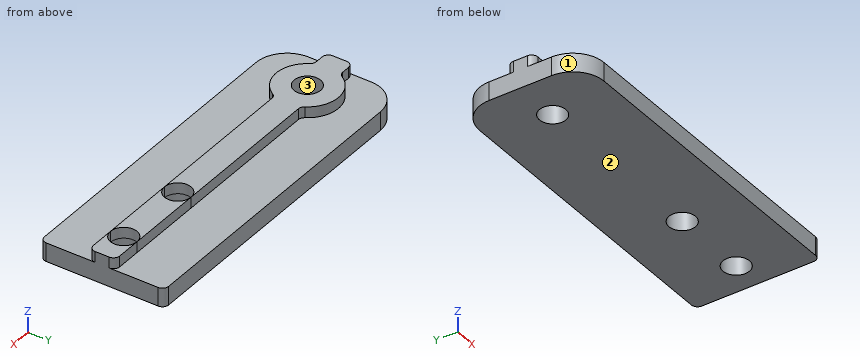
Autodesk Inventor part; units mm, degrees
ref_plane "YZ Plane" through (0, 0, 0) normal (1, 0, 0) x (0, 1, 0)
ref_plane "XZ Plane" through (0, 0, 0) normal (0, 1, 0) x (-1, 0, 0)
ref_plane "XY Plane" through (0, 0, 0) normal (0, 0, 1) x (1, 0, 0)
sketch "Szkic1" plane through (0, 0, 0) normal (0, 0, 1) x (1, 0, 0)
  line L0 (55, -20) -> (-55, -20)
  line L1 (-55, -20) -> (-55, 20)
  line L2 (-55, 20) -> (55, 20)
  line L3 (55, 20) -> (55, -20)
  line L4 (55, -20) -> (-55, 20) construction
  line L5 (-55, -20) -> (55, 20) construction
  line L6 (-55, 0) -> (55, 0) construction
  line L7 (-55, -4.25) -> (55, -4.25)
  line L8 (55, -4.25) -> (55, 4.25)
  line L9 (55, 4.25) -> (-55, 4.25)
  line L10 (-55, 4.25) -> (-55, -4.25)
  line L11 (-55, -4.25) -> (55, 4.25) construction
  line L12 (55, -4.25) -> (-55, 4.25) construction
  circle A0 centre (-40, 0) radius 10
  point P0 (0, 0)
  point P1 (0, 0)
  point P2 (-40, 0)
  point P3 (20, 0)
  point P4 (45, 0)
  dimension "d1" = 40
  dimension "d4" = 8.5
  dimension "d9" = 15
  dimension "d12" = 10
  dimension "d31" = 95
  dimension "d32" = 25
  dimension "d33" = 20
extrude "Wyciągnięcie proste1" add sketch "Szkic1" against normal blind 6
extrude "Wyciągnięcie proste2" add sketch "Szkic1" along normal blind 3.5 contours L7 A0 L9 L3 | L1 L9 A0 L7 | A0 L7 | L7 A0 L9 | L9 A0
fillet "Zaokrąglenie1" radius 2 10 edges at (55, 4.25, 1.75) (55, -4.25, 1.75) (55, 20, -3) (55, -20, -3) (-55, -4.25, 1.75) (-55, 4.25, 1.75) (-49.0519, -4.25, 1.75) (-30.9481, -4.25, 1.75) (-30.9481, 4.25, 1.75) (-49.0519, 4.25, 1.75)
fillet "Zaokrąglenie2" radius 10 2 edges at (-55, -20, -3) (-55, 20, -3)
hole "Otwór1" at (-40, 0, 0) at (20, 0, 0) at (45, 0, 0) direction (0, 0, -1) diameter 8.5 end through all
hole "Otwór2" at (45, 0, 0) at (20, 0, 0) at (-40, 0, 0) direction (0, 0, 1) diameter 8.5 end through all
properties part number "adapter_50mm"
Source: CAD feature listing. Evaluate the final solid. Frame: model axes, mm. Face numbers are marked on the shaded views. Give positions to 0.01 mm unless a question says otherwise; leave off trailing zeros. Order: outer loops, then holes, each group sorted by start corner. A loop starts at its lowest first (then second) coordinate and runs counter-clockwise, first axis right, second up. Notation, with made-up numbers: (45.5, 22.5) -> (96.5, 22.5) arc R12 ccw to (96.5, 34.5) -> close; hole circle Ø9 at (-20.75, -19). An arc over 180 degrees is marked (long way). Use a Markdown table: item, result.
Q1. Section D-D (y = 8). Return the cut outline in (x, z).
A:
| item | result |
|---|---|
| outline | (-55, -6) -> (55, -6) -> (55, 0) -> (-34, 0) -> (-34, 3.5) -> (-46, 3.5) -> (-46, 0) -> (-55, 0) -> close |
Q2. First-contact query: P1, Ø5.5, axis at x = -17, y = 10, coming from the +Z side; P2, Ø1, axis at x = 48.5, z = 2, coming from the +Y side; P3, Ø1.8, axis at x = 37.5, z = 2, coming from the -Y side; P4, Ø2, axis at y = 16, z = 2.5, coming from the +X side. Flat tips, straight axial feed; report the tip coordinate or a pass-through.
A:
| item | result |
|---|---|
| P1 | z = 0 |
| P2 | y = 4.25 |
| P3 | y = -4.25 |
| P4 | through |
Q3. Pull-direction query (Y, two-part tool) for the marked faces 1, 2 and 3; classes: +Y half, -Y half, draft (parallel to the pull), parting line (faces both ways), or undercut.
A:
| item | result |
|---|---|
| face 1 | -Y half |
| face 2 | draft |
| face 3 | undercut |
Q4. Section B-B (x = -40). Return the cut outline in (y, z).
A:
| item | result |
|---|---|
| outline | (-20, -6) -> (-4.25, -6) -> (-4.25, 3.5) -> (-10, 3.5) -> (-10, 0) -> (-20, 0) -> close; (4.25, -6) -> (20, -6) -> (20, 0) -> (10, 0) -> (10, 3.5) -> (4.25, 3.5) -> close |
Q5. Material intervals for line 1 (X direction, y = 0, z = -3); line 2 (Y direction, x = 45, z = -3.1); line 3 (Y direction, x = -40, z = 0.25), sorted ascending. Write a range as [from, to].
A:
| item | result |
|---|---|
| line 1 | [-55, -44.25], [-35.75, 15.75], [24.25, 40.75], [49.25, 55] |
| line 2 | [-20, -4.25], [4.25, 20] |
| line 3 | [-10, -4.25], [4.25, 10] |
Q6. Section C-C (y = 0). Return the cut outline in (x, z), and give its area (3 significant figures).
A:
| item | result |
|---|---|
| outline | (-55, -6) -> (-44.25, -6) -> (-44.25, 3.5) -> (-55, 3.5) -> close; (-35.75, -6) -> (15.75, -6) -> (15.75, 3.5) -> (-35.75, 3.5) -> close; (24.25, -6) -> (40.75, -6) -> (40.75, 3.5) -> (24.25, 3.5) -> close; (49.25, -6) -> (55, -6) -> (55, 3.5) -> (49.25, 3.5) -> close |
| area | 803 mm^2 |
